Source: CAD feature listing. Evaluate the final solid. Frame: model axes, mm. Face numbers are marked on the shaded views. Round coordinates to 2 decimals unless told otherwise and drop trailing zeros. Order: outer loops, then holes, each group sorted by start corner. A loop starts at its lowest first (then second) coordinate and runs counter-clockwise, first axis right, second up.
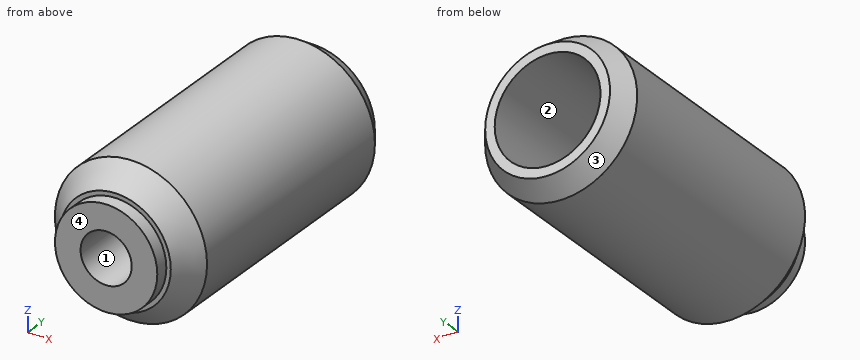
```python
from build123d import *

# Parameters (mm, degrees)
ESQUISSE1_R             = 11.15
BOSS_EXTRU_1_DEPTH      = 45.6
ESQUISSE2_R             = 7.75
ENL_V_MAT_EXTRU_1_DEPTH = 33
ESQUISSE3_R             = 11.15
ESQUISSE3_R_2           = 7.5
ENL_V_MAT_EXTRU_2_DEPTH = 2
ESQUISSE4_R             = 3.75
ENL_V_MAT_EXTRU_3_DEPTH = 46.6
CHANFREIN1_SIZE         = 3
CHANFREIN1_SIZE2        = 2
CHANFREIN2_SIZE         = 3.5
CHANFREIN2_SIZE2        = 3


with BuildPart() as part:
    # Esquisse1 → Boss.-Extru.1 (new body)
    with BuildSketch(Plane(origin=(0, 0, 0), x_dir=(1, 0, 0), z_dir=(0, 1, 0))):
        Circle(ESQUISSE1_R)
    extrude(amount=BOSS_EXTRU_1_DEPTH)

    # Esquisse2 → Enlèv. mat.-Extru.1 (cut)
    with BuildSketch(Plane(origin=(0, 45.6, 0), x_dir=(1, 0, 0), z_dir=(0, 1, 0))):
        Circle(ESQUISSE2_R)
    extrude(amount=-ENL_V_MAT_EXTRU_1_DEPTH, mode=Mode.SUBTRACT)

    # Esquisse3 → Enlèv. mat.-Extru.2 (cut)
    with BuildSketch(Plane.XZ):
        Circle(ESQUISSE3_R)
        Circle(ESQUISSE3_R_2, mode=Mode.SUBTRACT)
    extrude(amount=-ENL_V_MAT_EXTRU_2_DEPTH, mode=Mode.SUBTRACT)

    # Esquisse4 → Enlèv. mat.-Extru.3 (cut, through all)
    with BuildSketch(Plane.XZ):
        Circle(ESQUISSE4_R)
    extrude(amount=-ENL_V_MAT_EXTRU_3_DEPTH, mode=Mode.SUBTRACT)

    # Chanfrein1
    chanfrein1_edges = [part.edges().sort_by_distance(p)[0] for p in [
        (-11.15, 45.6, 0),
    ]]
    chanfrein1_side = [part.faces().sort_by_distance(p)[0] for p in [
        (-11.15, 23.8, 0),
    ]]
    chamfer(chanfrein1_edges, length=CHANFREIN1_SIZE, length2=CHANFREIN1_SIZE2, reference=chanfrein1_side[0])

    # Chanfrein2
    chanfrein2_edges = [part.edges().sort_by_distance(p)[0] for p in [
        (-11.15, 2, 0),
    ]]
    chanfrein2_side = [part.faces().sort_by_distance(p)[0] for p in [
        (-11.15, 22.3, 0),
    ]]
    chamfer(chanfrein2_edges, length=CHANFREIN2_SIZE, length2=CHANFREIN2_SIZE2, reference=chanfrein2_side[0])


solid = part.part
```
1. First-contact query: pin 1 (5 mm diameter, centred on y = 7.5, z = 5.5, fed in from +X); pin 2 (6 mm diameter, centred on x = 3.5, y = 38.5, fed in from +Z); pin 3 (4 mm diameter, centred on y = 38, z = -4, fed in from +X). Flat tips, straight axial feed; report the tip coordinate or a pass-through.
2. Section B-B on z = 0. Return loops of the section in (x, y), plus the area to 3 significant figures.
3. Pull-direction query (Z, two-part tool) for the marked faces 1, 2, 3 and 4; classes: released by +Z, released by -Z, zero draft, split by the parting line, or undercut.
4. Section D-D on y = 33. Return loops of the section in (x, z), plus the area to 3 significant figures.
5. Section A-A on x = 0. Return loops of the section in (y, z).
6. Section C-C on y = 7.5. Return loops of the section in (x, z).
7. Line query: line 1 along Z through (x, y) = (0, 9); line 2 along X through (y, z) = (25, 0); line 3 along Y through (x, z) = (-5.75, 5.75). Output: solid intervals per line, ascending.
Result:
1. pin 1: stops at x = 10.74
1. pin 2: stops at z = 11.14
1. pin 3: stops at x = 10.97
2. outline: (-11.15, 5.5) - (-8.15, 2) - (-7.5, 2) - (-7.5, 0) - (-3.75, 0) - (-3.75, 12.6) - (-7.75, 12.6) - (-7.75, 45.6) - (-9.15, 45.6) - (-11.15, 42.6) - close; (3.75, 0) - (7.5, 0) - (7.5, 2) - (8.15, 2) - (11.15, 5.5) - (11.15, 42.6) - (9.15, 45.6) - (7.75, 45.6) - (7.75, 12.6) - (3.75, 12.6) - close
2. area: 380 mm2
3. face 1: undercut
3. face 2: undercut
3. face 3: split by the parting line
3. face 4: zero draft
4. outline: circle Ø22.3 at (0, 0); hole circle Ø15.5 at (0, 0)
4. area: 202 mm2
5. outline: (0, -7.5) - (2, -7.5) - (2, -8.15) - (5.5, -11.15) - (42.6, -11.15) - (45.6, -9.15) - (45.6, -7.75) - (12.6, -7.75) - (12.6, -3.75) - (0, -3.75) - close; (0, 3.75) - (12.6, 3.75) - (12.6, 7.75) - (45.6, 7.75) - (45.6, 9.15) - (42.6, 11.15) - (5.5, 11.15) - (2, 8.15) - (2, 7.5) - (0, 7.5) - close
6. outline: circle Ø22.3 at (0, 0); hole circle Ø7.5 at (0, 0)
7. line 1: z = -11.15 to -3.75, 3.75 to 11.15
7. line 2: x = -11.15 to -7.75, 7.75 to 11.15
7. line 3: y = 2 to 45.6
